CAD build for the part. Positions are in the model's coordinates, mm. Face numbers are marked on the shaded views. A direction names the side the tool comes from. Round coordinates to 2 decimals unless told otherwise and drop trailing zeros. Write each loop counter-clockwise with the first axis right and the second up, starting at its lowest first coordinate (ties: lowest second). Pieces come first, ordered by that corner, then holes. Notation, with made-up numbers: M -4,18.25 L 37,18.25 A27 ccw 37,36.25 Z; hole C 25,42.25 d9. An arc over 180 degrees is marked long. Write each question's results on one line, items separated by ' | '. Start each with the question number.
```python
from build123d import *

# Parameters (mm, degrees)
F1_DEPTH = 1.6256
F3_DEPTH = 2.3876
F5_R     = 7.874
F6_DEPTH = 1.524


with BuildPart() as f1:
    # F0 (on Top) → F1 (new body)
    with BuildSketch(Plane.XY):
        Polygon((-22.8219, -39.52869), (22.8219, -39.52869), (45.6438, 0), (22.8219, 39.52869), (-22.8219, 39.52869), (-45.6438, 0), align=None)
    extrude(amount=F1_DEPTH)

    # F2 (on Top) → F3 (join)
    with BuildSketch(Plane.XY):
        Polygon((-20.006278, -34.65189), (20.006278, -34.65189), (40.012556, 0), (20.006278, 34.65189), (-20.006278, 34.65189), (-40.012556, 0), align=None)
    extrude(amount=F3_DEPTH)

    # F5 (on face) → F6 (cut)
    with BuildSketch(Plane.XY.offset(2.3876)):
        with Locations((22.8219, -39.52869)):
            Circle(F5_R)
        with Locations((45.6438, 0)):
            Circle(F5_R)
        with Locations((22.8219, 39.52869)):
            Circle(F5_R)
        with Locations((-22.8219, 39.52869)):
            Circle(F5_R)
        with Locations((-45.6438, 0)):
            Circle(F5_R)
        with Locations((-22.8219, -39.52869)):
            Circle(F5_R)
    extrude(amount=-F6_DEPTH, mode=Mode.SUBTRACT)


solid = f1.part
```
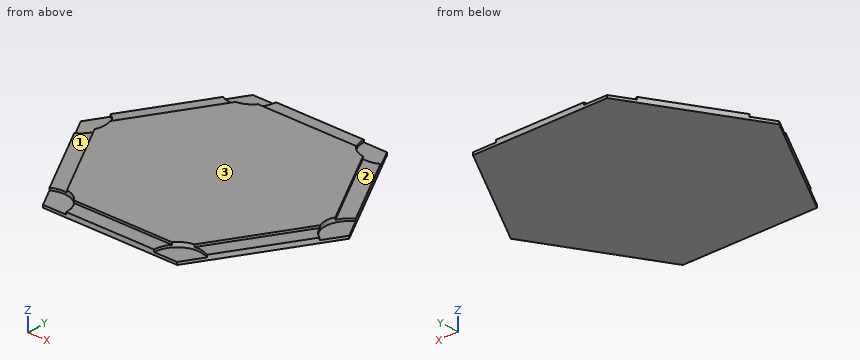
1) Drop flat-ended pins along their axis: pin 1 Ø2.5 at (x, y) = (42, 1.5) entering from +Z; pin 2 Ø1 at (y, z) = (-8, 1.5) entering from +X; pin 3 Ø1.5 at (x, y) = (-1.5, -36.5) entering from +Z. Give the stop position or say it passes through.
2) Wall check: line 1 along X through (y, z) = (32.5, 0.9); line 2 along Z through (x, y) = (-19.5, -33); line 3 along Z through (x, y) = (37.5, -5). Give the ranges that are in metal, low to high. Write a range as from..to.
3) Saw through at B-B, the plane y = 14. Write the cut outline in (x, z), plus the area to 3 significant figures.
4) Saw through at A-A, the plane x = -9.5. Write the cut outline in (y, z).
5) 3-axis set-ups, long thin cutter, end or side, ignore diameter. For the marked faces 1, 2 and 3: which of +Z, -Z, +X, -X, +Y, -Y reach the whole face in a straight line?
Filled sheet:
1) pin 1: stops at z = 0.86 | pin 2: stops at x = 41.31 | pin 3: stops at z = 1.63
2) line 1: x = -26.88..-26.37, -19.27..19.27, 26.37..26.88 | line 2: z = 0..0.86 | line 3: z = 0..1.63
3) outline: M -37.56,0 L 37.56,0 L 37.56,1.63 L 31.93,1.63 L 31.93,2.39 L -31.93,2.39 L -31.93,1.63 L -37.56,1.63 Z | area: 171 mm^2
4) outline: M -39.53,0 L 39.53,0 L 39.53,1.63 L 34.65,1.63 L 34.65,2.39 L -34.65,2.39 L -34.65,1.63 L -39.53,1.63 Z
5) face 1: +Z, -X, -Y | face 2: +Z, +X, +Y | face 3: +Z, +X, -X, +Y, -Y
